CAD build for the part. Positions are in the model's coordinates, mm. Face numbers are marked on the shaded views. Coordinates: 2 decimals unless noted, no trailing zeros. Write each loop counter-clockwise with the first axis right and the second up, starting at its lowest first coordinate (ties: lowest second). Pieces come first, ordered by that corner, then holes. Notation, with made-up numbers: (44, -24.75) - (80, -24.75) arc R16 ccw to (80, -18.75) - close; hole circle Ø1 at (-31, 88.5). An arc over 180 degrees is marked (long way). Answer in a Markdown table with one row per item. Add a question column.
Q1. Pin check, flat tips, straight feed: pin 1 (1.5 mm diameter, centred on x = 9.5, y = 9, fed in from -Z); pin 2 (2 mm diameter, centred on x = 12, z = 22.5, fed in from +Y); pin 3 (10 mm diameter, centred on y = 7.5, z = 45, fed in from +X). Stop position of each tip, or through.
Q2. Band-saw the part on A-A (y = 0). List the corners of the cut face in (x, z).
Q3. Band-saw the part on C-C (z = 106.5). List the corners of the cut face in (x, y).
Q4. Two-plate mould, pull along X, no slides. Class the marked faces 1 and 2: +X half, -X half, draft (parallel to the pull), parting line (faces both ways), or undercut.
Q5. Drill centre lines: line 1 along Y through (x, z) = (0, 83); line 2 along Y through (x, z) = (7.5, 24.5); line 3 along X through (y, z) = (-8.5, 16). Where is each one in solid material? Low to high. Write a range as from..to.
```python
from build123d import *

# Parameters (mm, degrees)
F0_R     = 16
F0_R_2   = 11
F1_DEPTH = 125


# Not quite as in the source:
# - a fillet or chamfer that OpenCascade refuses, or shapes differently, is made with other operations: its cross-section is extruded or revolved along the edge and cut away or added


with BuildPart() as f1:
    # F0 (on Top) → F1 (new body)
    with BuildSketch(Plane.XY):
        Circle(F0_R)
        Circle(F0_R_2, mode=Mode.SUBTRACT)
    extrude(amount=F1_DEPTH)

    # F2: fillet of radius 5.08 on 1 edges, made by hand

    # F2_s1 → F2_t2 (revolve, cut)
    with BuildSketch(Plane.XZ):
        with BuildLine():
            ThreePointArc((16, 119.92), (14.5121024484, 123.5121024484), (10.92, 125))
            Line((10.92, 125), (16, 125))
            Line((16, 125), (16, 119.92))
        make_face()
    revolve(axis=Axis((0, 0, 125), (0, 0, 1)), mode=Mode.SUBTRACT)

    # F3: fillet of radius 5.08 on 1 edges, made by hand

    # F3_s1 → F3_t2 (revolve, cut)
    with BuildSketch(Plane.XZ):
        with BuildLine():
            ThreePointArc((16, 5.08), (14.5121024484, 1.4878975516), (10.92, 0))
            Line((10.92, 0), (16, 0))
            Line((16, 0), (16, 5.08))
        make_face()
    revolve(axis=Axis((0, 0, 0), (0, 0, 1)), mode=Mode.SUBTRACT)


solid = f1.part
```
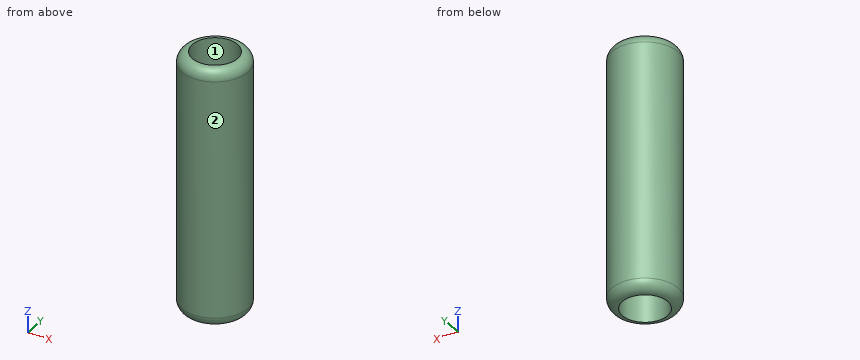
Checked values:
| question | item | result |
|---|---|---|
| 1 | pin 1 | stops at z = 0.2 |
| 1 | pin 2 | stops at y = 11.62 |
| 1 | pin 3 | stops at x = 15.8 |
| 2 | outline | (-16, 5.08) arc R5.08 ccw to (-11, 0) - (-11, 125) arc R5.08 ccw to (-16, 119.92) - close; (11, 0) arc R5.08 ccw to (16, 5.08) - (16, 119.92) arc R5.08 ccw to (11, 125) - close |
| 3 | outline | circle Ø32 at (0, 0); hole circle Ø22 at (0, 0) |
| 4 | face 1 | undercut |
| 4 | face 2 | parting line |
| 5 | line 1 | y = -16..-11, 11..16 |
| 5 | line 2 | y = -14.13..-8.05, 8.05..14.13 |
| 5 | line 3 | x = -13.56..-6.98, 6.98..13.56 |
